Verification items for the finished model (mm, model axes). A direction names the side the tool comes from. Coordinates: 2 decimals unless noted, no trailing zeros. Loops run counter-clockwise (first coordinate to the right, second up) from the corner with the lowest first, then second, coordinate; pieces in that order, holes last. Notation, with made-up numbers: (53.5, 30) -> (91.5, 30) arc R20 ccw to (91.5, 58) -> close; hole circle Ø1 at (81.5, 2.5). An arc over 180 degrees is marked (long way). Answer as a JSON object with one key per item and string values. Group by question number.
Q1. Cross-section at C-C on x = -24.5. Record the boundary of the cut face in (y, z), and give its area (3 significant figures).
Q2. Cross-section at B-B on y = 1.4. Give the number of separate pieces and of enclosed holes in the cut face, and give its area (3 significant figures).
Q3. Release check for a two-part mould opening along X. For faces 1 (the cylindrical face through (-38.824, 2.692, -21.177)), 2 (the flat face through (-10, 0, -9)), 3 (the cylindrical face through (-0.69, 2.69, 3.1)), 4 (the cylindrical face through (-39.932, 2.692, -29.787)) record: released by +X, released by -X, zero draft, split by the parting line, or undercut.
Q4. Cross-section at D-D on z = 5.5. Record the boundary of the cut face in (x, y), and give its area (3 significant figures).
Q5. Cross-section at A-A on x = 0. Record the boundary of the cut face in (y, z) (3 decimals).
Q6. Scan lines: L1, parallel to X at y = 1.1, z = 0 (3 decimals); L2, parallel to Z at x = -19.5, y = 1.85; L3, parallel to X at y = 3.1, z = -13.5. Record each from-to range of solid material in increasing order.
Q7. Gauge pin test, flat ends, axial feed: pin 1 Ø2 at (y, z) = (3, -10.5) entering from +X; pin 2 Ø1.5 at (y, z) = (5, -3) entering from -X; pin 3 Ø3 at (y, z) = (1, -24) entering from -X; pin 4 Ø4 at (x, z) = (0, 0) entering from +Y. Record the tip position at first contact, or that the pin passes through.
Q8. Set-up check for faces 5 (the cylindrical face through (-20.042, 2.692, -13.516)), 6 (the flat face through (-41.164, 2.692, -15.693)): record each of +Z, -Z, +X, -X, +Y, -Y from which the full face is reachable in a straight line by a thin tool's end or side.
```python
from build123d import *

# Parameters (mm, degrees)
SKETCH1_R           = 1.778
SKETCH1_R_2         = 3.175
BOSS_EXTRUDE1_DEPTH = 5.461


with BuildPart() as part:
    # Sketch1 → Boss-Extrude1 (new body)
    with BuildSketch(Plane(origin=(0, 0, 0), x_dir=(1, 0, 0), z_dir=(0, 1, 0))):
        with BuildLine():
            Line((-38.770225031, 16.757963615), (-43.625448569, 14.598747375))
            ThreePointArc((-43.625448569, 14.598747375), (-45.155674622, 14.559326862), (-46.265582353, 15.613485569))
            Line((-46.265582353, 15.613485569), (-47.282683039, 17.900542834))
            ThreePointArc((-47.282683039, 17.900542834), (-47.541465806, 19.100109045), (-47.298283286, 20.302934833))
            ThreePointArc((-47.298283286, 20.302934833), (-45.865213893, 23.360627542), (-44.234733225, 26.317772344))
            ThreePointArc((-44.234733225, 26.317772344), (-39.855484626, 29.811728531), (-34.259632886, 29.543416329))
            Line((-34.259632886, 29.543416329), (5.363638877, 12.388760148))
            ThreePointArc((5.363638877, 12.388760148), (7.44200849, -11.263503435), (-13.499793526, -0.074664302))
            Line((-13.499793526, -0.074664302), (-36.286855081, 16.495885282))
            ThreePointArc((-36.286855081, 16.495885282), (-37.403602541, 17.810792136), (-38.770225031, 16.757963615))
        make_face()
        with Locations((-20.862458922, 15.093717491)):
            Circle(SKETCH1_R, mode=Mode.SUBTRACT)
        Circle(SKETCH1_R_2, mode=Mode.SUBTRACT)
        with Locations((-37.413253893, 22.259284205)):
            Circle(SKETCH1_R, mode=Mode.SUBTRACT)
    extrude(amount=BOSS_EXTRUDE1_DEPTH)


solid = part.part
```
Computed values:
{
 "1": {"outline": "(0, -25.32) -> (5.46, -25.32) -> (5.46, -7.92) -> (0, -7.92) -> close", "area": "95.0 mm²"},
 "2": {"separate pieces": "1", "enclosed holes": "3", "area": "1,140 mm²"},
 "3": {"face 1": "undercut", "face 2": "zero draft", "face 3": "undercut", "face 4": "split by the parting line"},
 "4": {"outline": "(-12.33, 0) -> (12.33, 0) -> (12.33, 5.46) -> (-12.33, 5.46) -> close", "area": "135 mm²"},
 "5": {"outline": "(0, -14.711) -> (5.461, -14.711) -> (5.461, -3.175) -> (0, -3.175) -> close; (0, 3.175) -> (5.461, 3.175) -> (5.461, 13.5) -> (0, 13.5) -> close"},
 "6": {"L1": "x = -13.602 to -3.175, 3.175 to 13.5", "L2": "z = -23.15 to -16.24, -13.95 to -4.29", "L3": "x = -32.17 to -21.65, -20.07 to 2.8"},
 "7": {"pin 1": "stops at x = 9.59", "pin 2": "stops at x = -18.76", "pin 3": "stops at x = -46.29", "pin 4": "passes through"},
 "8": {"face 5": "+Y, -Y", "face 6": "+Z, +Y, -Y"}
}
